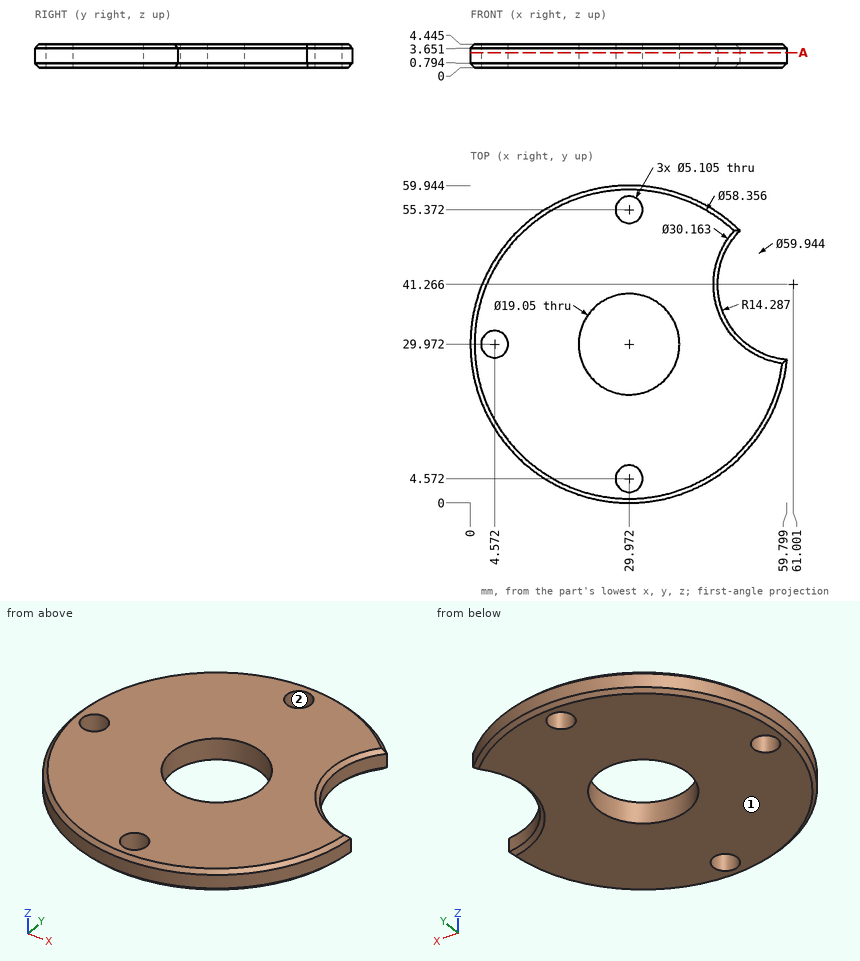
Geometry: see drawing. Coordinates: mm, zero at the bounding-box minimum. Round coordinates to 2 decimals unless told otherwise and drop trailing zeros. Use a Markdown table: item, result. Add a question column.
1. Line query: line 1 (Y direction, x = 30.5, z = 1.9) (1 decimal); line 2 (X direction, y = 57, z = 3.2) (1 decimal); line 3 (X direction, y = 43.5, z = 1.2) (1 decimal). Output: solid intervals per line, ascending.
2. Contact query for flat-ended pins moving along their axis: P1, Ø1, axis at x = 23, z = 1, coming from the +Y side; P2, Ø4, axis at x = 4.572, y = 29.972, coming from the -Z side; P3, Ø1.5, axis at x = 11.5, z = 3.5, coming from the -Y side. Output: stop coordinate, or through.
3. Mould query, pull axis X, two halves, no side actions, for the marked faces 1 and 2. Classes: pulls with the +X half, pulls with the -X half, needs draft (parallel to the pull), parting line crosses it, or undercut.
4. Section query A-A on z = 2.8. Give the number of separate pieces and of enclosed holes in the cut face, then the cut area to 3 significant figures.
Reported:
| question | item | result |
|---|---|---|
| 1 | line 1 | y = 0 to 2.1, 7.1 to 20.5, 39.5 to 52.9, 57.9 to 59.9 |
| 1 | line 2 | x = 17 to 28, 31.9 to 42.9 |
| 1 | line 3 | x = 3.2 to 46.9 |
| 2 | P1 | stops at y = 59.24 |
| 2 | P2 | passes through |
| 2 | P3 | stops at y = 5.8 |
| 3 | face 1 | needs draft |
| 3 | face 2 | undercut |
| 4 | separate pieces | 1 |
| 4 | enclosed holes | 4 |
| 4 | area | 2,270 mm² |
